from build123d import *

# Parameters (mm, degrees)
SKETCH1_R                   = 25.9
SKETCH1_R_2                 = 12.5
BOSS_EXTRUDE1_DEPTH         = 6.35
F_1_4_CLEARANCE_HOLE1_D     = 6.7564
F_1_4_CLEARANCE_HOLE1_DEPTH = 19.53
F_1_4_CLEARANCE_HOLE1_TIP   = 2.029827343
FILLET1_R                   = 10
FILLET2_R                   = 3


with BuildPart() as part:
    # Sketch1 → Boss-Extrude1 (new body)
    with BuildSketch(Plane(origin=(0, 0, 0), x_dir=(1, 0, 0), z_dir=(0, 1, 0))):
        with BuildLine():
            Line((-64.5, 160), (-19, 160))
            Line((-19, 160), (-19, 179))
            ThreePointArc((-19, 179), (0, 198), (19, 179))
            Line((19, 179), (19, 160))
            Line((19, 160), (64.5, 160))
            Line((64.5, 160), (64.5, -166))
            Line((64.5, -166), (-64.5, -166))
            Line((-64.5, -166), (-64.5, 160))
        make_face()
        with Locations(Location((0, -130, 0), (0, 0, 270))):  # turned: the seam where the file's is
            Circle(SKETCH1_R, mode=Mode.SUBTRACT)
        with Locations(Location((0, 179, 0), (0, 0, 270))):  # turned: the seam where the file's is
            Circle(SKETCH1_R_2, mode=Mode.SUBTRACT)
    extrude(amount=BOSS_EXTRUDE1_DEPTH)

    # 1/4 Clearance Hole1
    with Locations(Plane(origin=(0, 6.35, 0), x_dir=(1, 0, 0), z_dir=(0, 1, 0))):
        with Locations((-39.5, 135), (39.5, 135), (39.5, -135), (-39.5, -135)):
            Hole(F_1_4_CLEARANCE_HOLE1_D / 2, depth=F_1_4_CLEARANCE_HOLE1_DEPTH)
            with Locations((0, 0, -(F_1_4_CLEARANCE_HOLE1_DEPTH + F_1_4_CLEARANCE_HOLE1_TIP / 2))):  # 118° drill point
                Cone(0, F_1_4_CLEARANCE_HOLE1_D / 2, F_1_4_CLEARANCE_HOLE1_TIP, mode=Mode.SUBTRACT)

    # Fillet1
    fillet1_edges = [part.edges().sort_by_distance(p)[0] for p in [
        (-19, 3.175, -160),
        (19, 3.175, -160),
    ]]
    fillet(fillet1_edges, radius=FILLET1_R)

    # Fillet2
    fillet2_edges = [part.edges().sort_by_distance(p)[0] for p in [
        (64.5, 3.175, 166),
        (-64.5, 3.175, 166),
        (-64.5, 3.175, -160),
        (64.5, 3.175, -160),
    ]]
    fillet(fillet2_edges, radius=FILLET2_R)


solid = part.part
CAD build for the part. Positions are in the model's coordinates, mm. A direction names the side the tool comes from. Give positions to 0.01 mm unless a question says otherwise; leave off trailing zeros. Order: outer loops, then holes, each group sorted by start corner. A loop starts at its lowest first (then second) coordinate and runs counter-clockwise, first axis right, second up. Notation, with made-up numbers: (69, -14.75) -> (124, -14.75) arc R20 cw to (124, -9.75) -> close; hole circle Ø4 at (29, 71). An arc over 180 degrees is marked (long way). Return JSON: item names as keys, results as strings.
Q1. Which spindle directions (+Z, -Z, +X, -X, +Y, -Y) get a long thin tool onto all of the face, cutting with end or side? Do faces 5 (the face through (1.139, 3.131, 104.125)), 6 (the face through (45, 3, -160)), 7 (the face through (-45, 3, -160)). Say none if no direction does.
Working result:
{"face 5": "+Y, -Y", "face 6": "-Z, +X, +Y, -Y", "face 7": "-Z, -X, +Y, -Y"}
Q2. Saw through at D-D (z = 135). Write the cut outline in (x, y), then the cut area to 3 significant figures.
Working result:
{"outline": "(-64.5, 0) -> (-42.88, 0) -> (-42.88, 6.35) -> (-64.5, 6.35) -> close; (-36.12, 0) -> (-25.41, 0) -> (-25.41, 6.35) -> (-36.12, 6.35) -> close; (25.41, 0) -> (36.12, 0) -> (36.12, 6.35) -> (25.41, 6.35) -> close; (42.88, 0) -> (64.5, 0) -> (64.5, 6.35) -> (42.88, 6.35) -> close", "area": "411 mm²"}
Q3. Saw through at B-B (y = 1.5). Write the cut outline in (x, z), then the cut area to 3 significant figures.
Working result:
{"outline": "(-64.5, -157) arc R3 ccw to (-61.5, -160) -> (-29, -160) arc R10 cw to (-19, -170) -> (-19, -179) arc R19 ccw to (19, -179) -> (19, -170) arc R10 cw to (29, -160) -> (61.5, -160) arc R3 ccw to (64.5, -157) -> (64.5, 163) arc R3 ccw to (61.5, 166) -> (-61.5, 166) arc R3 ccw to (-64.5, 163) -> close; hole circle Ø6.76 at (-39.5, -135); hole circle Ø6.76 at (-39.5, 135); hole circle Ø51.8 at (0, 130); hole circle Ø25 at (0, -179); hole circle Ø6.76 at (39.5, -135); hole circle Ø6.76 at (39.5, 135)", "area": "40,600 mm²"}
Q4. Saw through at A-A (z = -135). Write the cut outline in (x, y), then the cut area to 3 significant figures.
Working result:
{"outline": "(-64.5, 0) -> (-42.88, 0) -> (-42.88, 6.35) -> (-64.5, 6.35) -> close; (-36.12, 0) -> (36.12, 0) -> (36.12, 6.35) -> (-36.12, 6.35) -> close; (42.88, 0) -> (64.5, 0) -> (64.5, 6.35) -> (42.88, 6.35) -> close", "area": "733 mm²"}
Q5. Flat gauge pins, fed straight in: pin 1 (3 mm diameter, centred on x = 40, y = 3, fed in from -Z); pin 2 (3 mm diameter, centred on y = 2, z = -176.5, fed in from +X); pin 3 (1.5 mm diameter, centred on x = 17, y = 4, fed in from -Z). Where does each tip first touch, or does it go through?
Working result:
{"pin 1": "z = -160", "pin 2": "x = 19", "pin 3": "z = -188.85"}
Q6. Saw through at C-C (x = 39.5). Write the cut outline in (y, z).
Working result:
{"outline": "(0, -160) -> (6.35, -160) -> (6.35, -138.38) -> (0, -138.38) -> close; (0, -131.62) -> (6.35, -131.62) -> (6.35, 131.62) -> (0, 131.62) -> close; (0, 138.38) -> (6.35, 138.38) -> (6.35, 166) -> (0, 166) -> close"}
Q7. Mould opens along Z. For faces 1 (the face through (40.23, 3.13, -131.7)), 2 (the face through (40.23, 3.13, 138.3)), 3 (the face through (0, 3, -198)), 4 (the face through (64.5, 3, 1)) say: pulls with the +Z half, pulls with the -Z half, needs draft (parallel to the pull), parting line crosses it, or undercut.
Working result:
{"face 1": "undercut", "face 2": "undercut", "face 3": "pulls with the -Z half", "face 4": "needs draft"}
Q8. Drill centre lines: line 1 (Z direction, x = 39.5, y = 1.75); line 2 (X direction, y = 3, z = -135); line 3 (Z direction, x = 0.5, y = 2). Where is each one in solid material? Low to high.
Working result:
{"line 1": "-160 to -138.38, -131.62 to 131.62, 138.38 to 166", "line 2": "-64.5 to -42.88, -36.12 to 36.12, 42.88 to 64.5", "line 3": "-197.99 to -191.49, -166.51 to 104.1, 155.9 to 166"}
